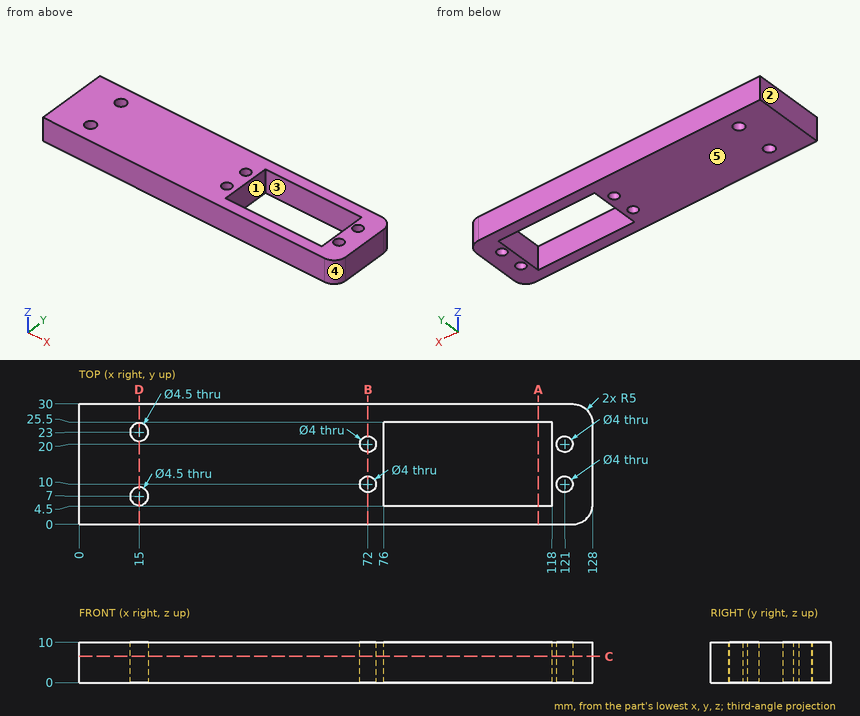
Verification items for this drawing (mm, ordinates from the low corner). A direction names the side the tool comes from. Coordinates: 2 decimals unless noted, no trailing zeros. Write each loop counter-clockwise with the first axis right and the second up, starting at its lowest first coordinate (ties: lowest second). Pieces come first, ordered by that corner, then holes. Notation, with made-up numbers: (-6, -31) -> (44, -31) arc R17 cw to (44, -5) -> close; hole circle Ø5 at (81.25, 26.25). An arc over 180 degrees is marked (long way). One line per item, written item: value. Start each with the question number.
Q1. Mould release check, pull along Y, two halves, no side actions. Record for the marked faces 3, 4 and 5: pulls with the +Y half, pulls with the -Y half, needs draft (parallel to the pull), parting line crosses it, or undercut.
Q2. Cross-section at A-A on x = 114.5. Enter the section's corners in (y, z), and give its area (3 significant figures).
Q3. Thickness scan on L1, parallel to Y at x = 121, z = 7; L2, parallel to X at y = 19.75, z = 6; L3, parallel to Y at x = 15, z = 6.5. Record the ranges inside material, lowest first. Write a range as from..to.
Q4. Go/stop test with a flat-tipped pin: P1, Ø3, axis at x = 72, y = 10, coming from the +Z side. Record where the tip stops, or that it passes through.
Q5. Cross-section at C-C on z = 6.5. Enter the section's corners in (x, y).
Q6. Cross-section at D-D on x = 15. Enter the section's corners in (y, z).
Q7. Access from +Z, -Z, +X, -X, +Y, -Y to the whole of each face (thin tool, end or side, straight path). Record for the marked faces 1 and 2.
Q8. Cross-section at B-B on x = 72. Enter the section's corners in (y, z), and give its area (3 significant figures).
Checked values:
1. face 3: undercut
1. face 4: pulls with the -Y half
1. face 5: needs draft
2. outline: (0, 0) -> (4.5, 0) -> (4.5, 10) -> (0, 10) -> close; (25.5, 0) -> (30, 0) -> (30, 10) -> (25.5, 10) -> close
2. area: 90.0 mm²
3. L1: y = 0..8, 12..18, 22..30
3. L2: x = 0..70.02, 73.98..76, 118..119.02, 122.98..128
3. L3: y = 0..4.75, 9.25..20.75, 25.25..30
4. P1: passes through
5. outline: (0, 0) -> (123, 0) arc R5 ccw to (128, 5) -> (128, 25) arc R5 ccw to (123, 30) -> (0, 30) -> close; hole circle Ø4.5 at (15, 7); hole circle Ø4.5 at (15, 23); hole circle Ø4 at (72, 10); hole circle Ø4 at (72, 20); hole (76, 4.5) -> (118, 4.5) -> (118, 25.5) -> (76, 25.5) -> close; hole circle Ø4 at (121, 10); hole circle Ø4 at (121, 20)
6. outline: (0, 0) -> (4.75, 0) -> (4.75, 10) -> (0, 10) -> close; (9.25, 0) -> (20.75, 0) -> (20.75, 10) -> (9.25, 10) -> close; (25.25, 0) -> (30, 0) -> (30, 10) -> (25.25, 10) -> close
7. face 1: +Z, -Z
7. face 2: +Z, -Z, -X, +Y, -Y
8. outline: (0, 0) -> (8, 0) -> (8, 10) -> (0, 10) -> close; (12, 0) -> (18, 0) -> (18, 10) -> (12, 10) -> close; (22, 0) -> (30, 0) -> (30, 10) -> (22, 10) -> close
8. area: 220 mm²
